Design review of the part built by this model. Coordinates are the model's own, in mm. Coordinates: 2 decimals unless noted, no trailing zeros. Write item = value, one per line.
```python
from build123d import *

# Parameters (mm, degrees)
BOX_W        = 115
BOX_H        = 25.4
BOX_DEPTH    = 1
SKETCH_R     = 2.5
POCKET_DEPTH = 5


with BuildPart() as part:
    # Box → Box (new body)
    with BuildSketch(Plane.XY):
        with Locations((57.5, 12.7)):
            Rectangle(BOX_W, BOX_H)
    extrude(amount=BOX_DEPTH)

    # Sketch (on Face6 of BaseFeature) → Pocket (cut)
    with BuildSketch(Plane.XY.offset(1)):
        with Locations((12.527164, 17.504574)):
            Circle(SKETCH_R)
        with Locations((22.523344, 17.5024)):
            Circle(SKETCH_R)
        with Locations((32.519524, 17.500226)):
            Circle(SKETCH_R)
        with Locations((42.515704, 17.498052)):
            Circle(SKETCH_R)
        with Locations((52.511884, 17.495878)):
            Circle(SKETCH_R)
        with Locations((62.508064, 17.493704)):
            Circle(SKETCH_R)
        with Locations((72.504244, 17.49153)):
            Circle(SKETCH_R)
        with Locations((82.500424, 17.489356)):
            Circle(SKETCH_R)
        with Locations((92.496604, 17.487182)):
            Circle(SKETCH_R)
        with Locations((102.492784, 17.485008)):
            Circle(SKETCH_R)
        with Locations((12.52499, 7.508394)):
            Circle(SKETCH_R)
        with Locations((22.52117, 7.50622)):
            Circle(SKETCH_R)
        with Locations((32.51735, 7.504046)):
            Circle(SKETCH_R)
        with Locations((42.51353, 7.501872)):
            Circle(SKETCH_R)
        with Locations((52.50971, 7.499698)):
            Circle(SKETCH_R)
        with Locations((62.50589, 7.497524)):
            Circle(SKETCH_R)
        with Locations((72.50207, 7.49535)):
            Circle(SKETCH_R)
        with Locations((82.49825, 7.493176)):
            Circle(SKETCH_R)
        with Locations((92.49443, 7.491002)):
            Circle(SKETCH_R)
        with Locations((102.49061, 7.488828)):
            Circle(SKETCH_R)
    extrude(amount=-POCKET_DEPTH, mode=Mode.SUBTRACT)


solid = part.part
```
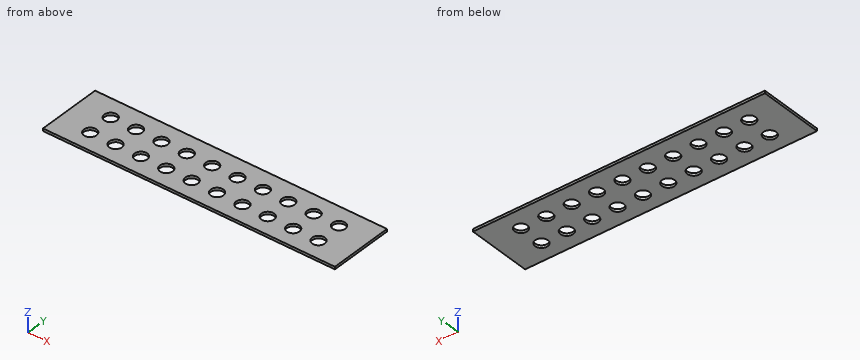
(1) Insertion check: pin 1 (3 mm diameter, centred on x = 72.5, y = 17.49, fed in from -Z). The pin has a flat end and moves straight along its axis. Give the tip position at first contact, or say it passes through.
Report:
pin_1 = through
(2) For L1, parallel to Y at x = 12.5, z = 0.45; L2, parallel to Y at x = 51.5, z = 0.7, list the stretches that pass through material, from the lowest coordinate up.
Report:
L1 = 0 to 5.01, 10.01 to 15, 20 to 25.4
L2 = 0 to 5.21, 9.79 to 15.21, 19.78 to 25.4
(3) We need section A-A (z = 0.3). Give the number of separate pieces and of enclosed holes in the cut face, and give its area (3 significant figures).
Report:
separate_pieces = 1
enclosed_holes = 20
area = 2,530 mm²
